from build123d import *

# Parameters (mm, degrees)
SKETCH1_R           = 3
BOSS_EXTRUDE1_DEPTH = 4
BOSS_EXTRUDE2_DEPTH = 14
CUT_EXTRUDE1_DEPTH  = 14
FILLET1_R           = 3


with BuildPart() as part:
    # Sketch1 → Boss-Extrude1 (new body)
    with BuildSketch(Plane.XY):
        with BuildLine():
            Line((-96.672208827, 8.599646064), (-96.672208827, 74.599646064))
            ThreePointArc((-96.672208827, 74.599646064), (-99.015354577, 80.256500313), (-104.672208827, 82.599646064))
            Line((-104.672208827, 82.599646064), (-105.672208827, 82.599646064))
            ThreePointArc((-105.672208827, 82.599646064), (-111.672208827, 88.599646064), (-105.672208827, 94.599646064))
            Line((-105.672208827, 94.599646064), (-104.672208827, 94.599646064))
            ThreePointArc((-104.672208827, 94.599646064), (-90.530073203, 88.741781688), (-84.672208827, 74.599646064))
            Line((-84.672208827, 74.599646064), (-84.672208827, 8.599646064))
            ThreePointArc((-84.672208827, 8.599646064), (-90.672208827, 2.599646064), (-96.672208827, 8.599646064))
        make_face()
        with Locations((-90.672208827, 68.599646064)):
            Circle(SKETCH1_R, mode=Mode.SUBTRACT)
        with Locations((-105.672208827, 88.599646064)):
            Circle(SKETCH1_R, mode=Mode.SUBTRACT)
        with BuildLine():
            Line((-92.672208827, 8.599646064), (-92.672208827, 18.599646064))
            ThreePointArc((-92.672208827, 18.599646064), (-90.672208827, 20.599646064), (-88.672208827, 18.599646064))
            Line((-88.672208827, 18.599646064), (-88.672208827, 8.599646064))
            ThreePointArc((-88.672208827, 8.599646064), (-90.672208827, 6.599646064), (-92.672208827, 8.599646064))
        make_face(mode=Mode.SUBTRACT)
    extrude(amount=BOSS_EXTRUDE1_DEPTH)

    # Sketch2 → Boss-Extrude2 (add)
    with BuildSketch(Plane(origin=(0, 0, 4), x_dir=(-1, 0, 0), z_dir=(0, 0, -1))):
        with BuildLine():
            Line((84.672208827, 28.599646064), (96.672208827, 28.599646064))
            Line((96.672208827, 28.599646064), (96.672208827, 8.599646064))
            ThreePointArc((96.672208827, 8.599646064), (90.672208827, 2.599646064), (84.672208827, 8.599646064))
            Line((84.672208827, 8.599646064), (84.672208827, 28.599646064))
        make_face()
        with BuildLine():
            Line((88.672208827, 8.599646064), (88.672208827, 18.599646064))
            ThreePointArc((88.672208827, 18.599646064), (90.672208827, 20.599646064), (92.672208827, 18.599646064))
            Line((92.672208827, 18.599646064), (92.672208827, 8.599646064))
            ThreePointArc((92.672208827, 8.599646064), (90.672208827, 6.599646064), (88.672208827, 8.599646064))
        make_face(mode=Mode.SUBTRACT)
    extrude(amount=-BOSS_EXTRUDE2_DEPTH)

    # Sketch3 → Cut-Extrude1 (cut)
    with BuildSketch(Plane(origin=(0, 0, 0), x_dir=(-1, 0, 0), z_dir=(0, 0, -1))):
        with BuildLine():
            Line((84.672208827, 8.599646064), (84.672208827, 24.599646064))
            Line((84.672208827, 24.599646064), (96.672208827, 24.599646064))
            Line((96.672208827, 24.599646064), (96.672208827, 8.599646064))
            ThreePointArc((96.672208827, 8.599646064), (90.672208827, 2.599646064), (84.672208827, 8.599646064))
        make_face()
        with BuildLine():
            Line((88.672208827, 8.599646064), (88.672208827, 18.599646064))
            ThreePointArc((88.672208827, 18.599646064), (90.672208827, 20.599646064), (92.672208827, 18.599646064))
            Line((92.672208827, 18.599646064), (92.672208827, 8.599646064))
            ThreePointArc((92.672208827, 8.599646064), (90.672208827, 6.599646064), (88.672208827, 8.599646064))
        make_face(mode=Mode.SUBTRACT)
    extrude(amount=-CUT_EXTRUDE1_DEPTH, mode=Mode.SUBTRACT)

    # Fillet1
    fillet1_edges = [part.edges().sort_by_distance(p)[0] for p in [
        (-90.672208827, 28.599646064, 4),
        (-90.672208827, 24.599646064, 0),
    ]]
    fillet(fillet1_edges, radius=FILLET1_R)


solid = part.part
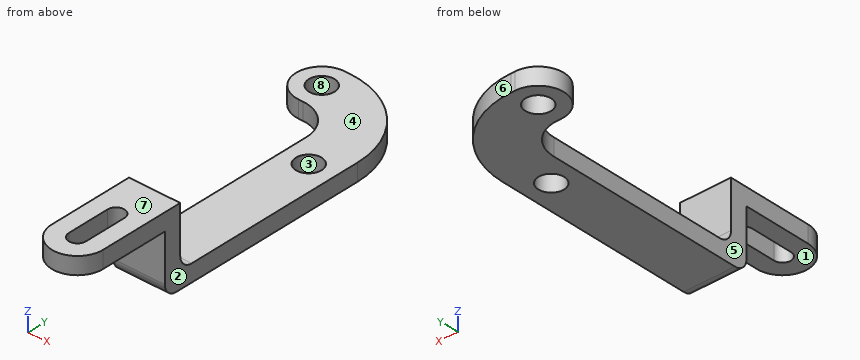
Check sheet for the modelled part. Datum: model origin and axes. Units: mm. Face numbers are marked on the shaded views. A direction names the side the tool comes from. Give positions to 0.01 mm unless a question says otherwise; leave off trailing zeros. Order: outer loops, then holes, each group sorted by start corner. A loop starts at its lowest first (then second) coordinate and runs counter-clockwise, first axis right, second up. Notation, with made-up numbers: M -33.75,52.5 L -9.75,52.5 A4 ccw -9.75,59.5 Z; hole C 44.25,26.25 d11. An arc over 180 degrees is marked long. Answer as CSV lines item,"result". Start each with the question number.
Item 1: Cross-section at C-C on x = -103.5. Enter the section's corners in (y, z).
Item 2: Cross-section at D-D on y = 33.5. Enter the section's corners in (x, z), plus the area to 3 significant figures.
Item 3: Cross-section at B-B on x = -89.5. Enter the section's corners in (y, z), plus the area to 3 significant figures.
Item 4: Tool access check on the marked faces 1, 2, 3, 4 and 5. Record the directions out of +Z, -Z, +X, -X, +Y, -Y that give a thin tool (end or side, any length) a straight path to the whole face; none if there is none.
Item 5: Gauge pin test, flat ends, axial feed: P1, Ø2, axis at x = -98, z = 16, coming from the -Y side; P2, Ø3, axis at y = 26.5, z = 4, coming from the -X side; P3, Ø13.5, axis at x = -95.5, y = 64, coming from the +Z side; P4, Ø9, axis at x = -93.5, z = 12.5, coming from the +Y side. Record the tip position at first contact, or that the pin passes through.
Item 6: Cross-section at A-A on y = 11. Enter the section's corners in (x, z), plus the area to 3 significant figures.
Item 7: Thickness scan on line 1 (Z direction, x = -96.5, y = 85); line 2 (Y direction, x = -92.75, z = 8); line 3 (X direction, y = 49, z = 2.5). Record the ranges inside material, lowest first. Write a range as [from, to].
Item 8: Mould release check, pull along Y, two halves, no side actions. Record for the marked faces 6, 7 and 8: +Y half, -Y half, draft (parallel to the pull), parting line (faces both ways), or undercut.
Established:
1,outline,"M 82.51,0 L 86.53,0 L 86.53,4 L 82.51,4 Z; M 90.67,0 L 94.57,0 L 94.57,4 L 90.67,4 Z"
2,outline,"M -96.67,0 L -84.67,0 L -84.67,4 L -96.67,4 Z"
2,area,"48.0 mm^2"
3,outline,"M 2.72,14 L 6.98,14 L 6.98,18 L 2.72,18 Z; M 20.22,14 L 24.6,14 L 24.6,3 A3 ccw 27.6,0 L 65.84,0 L 65.84,4 L 31.6,4 A3 cw 28.6,7 L 28.6,18 L 20.22,18 Z; M 71.36,0 L 87.63,0 L 87.63,4 L 71.36,4 Z"
3,area,"321 mm^2"
4,face 1,"-Z, +X, -X, -Y"
4,face 2,"+Z, -Z, +X, +Y, -Y"
4,face 3,"+Z, -Z"
4,face 4,"+Z, +X, -X, +Y"
4,face 5,"+Z, -Z, -X, -Y"
5,P1,"passes through"
5,P2,"stops at x = -96.67"
5,P3,"stops at z = 4"
5,P4,"stops at y = 28.6"
6,outline,"M -96.67,14 L -92.67,14 L -92.67,18 L -96.67,18 Z; M -88.67,14 L -84.67,14 L -84.67,18 L -88.67,18 Z"
6,area,"32.0 mm^2"
7,line 1,"z = [0, 4]"
7,line 2,"y = [24.6, 28.6]"
7,line 3,"x = [-96.67, -84.67]"
8,face 6,"+Y half"
8,face 7,"draft"
8,face 8,"undercut"
